Geometry: final body of the model. Coordinates: model frame, mm. A direction names the side the tool comes from. Round coordinates to 2 decimals unless told otherwise and drop trailing zeros. Loops run counter-clockwise (first coordinate to the right, second up) from the corner with the lowest first, then second, coordinate; pieces in that order, holes last. Notation, with made-up numbers: (-31, 37.5) -> (21, 37.5) arc R15 ccw to (21, 61.5) -> close; hole circle Ø3 at (29.5, -12). An arc over 180 degrees is marked (long way). Answer in a Markdown table with one row per item.
```python
from build123d import *

# Parameters (mm, degrees)
F0_R     = 35
F0_R_2   = 32.5
F1_DEPTH = 40
F2_START = 20
F0_R_3   = 12.5
F2_DEPTH = 20
F3_START = 39
F3_DEPTH = 61
F4_SIZE  = 20
F5_SIZE  = 18.99999
F6_START = 3
F0_R_4   = 40
F6_DEPTH = 12
F7_SIZE  = 4.99999
F8_DEPTH = 1.5


# Not quite as in the source:
# - a fillet or chamfer is up to 0.001 mm smaller than in the source, because OpenCascade refuses the exact size


with BuildPart() as f1:
    # F0 (on Top) → F1 (new body)
    with BuildSketch(Plane.XY):
        Circle(F0_R)
        Circle(F0_R_2, mode=Mode.SUBTRACT)
    extrude(amount=F1_DEPTH)

    # F0 (on Top) → F2 (join)
    with BuildSketch(Plane.XY.offset(F2_START)):
        Circle(F0_R_2)
        Circle(F0_R_3, mode=Mode.SUBTRACT)
    extrude(amount=F2_DEPTH)

    # F0 (on Top) → F3 (join)
    with BuildSketch(Plane.XY.offset(F3_START)):
        Circle(F0_R_3)
    extrude(amount=F3_DEPTH)

    # F4
    f4_edges = [f1.edges().sort_by_distance(p)[0] for p in [
        (-35, 0, 40),
    ]]
    chamfer(f4_edges, length=F4_SIZE)

    # F5 (size 19 in the source; OpenCascade refuses exactly that, so slightly less here)
    f5_edges = [f1.edges().sort_by_distance(p)[0] for p in [
        (-12.5, 0, 20),
    ]]
    chamfer(f5_edges, length=F5_SIZE)

    # F0 (on Top) → F6 (join)
    with BuildSketch(Plane.XY.offset(F6_START)):
        Circle(F0_R_4)
        Circle(F0_R, mode=Mode.SUBTRACT)
    extrude(amount=F6_DEPTH)

    # F7 (size 5 in the source; OpenCascade refuses exactly that, so slightly less here)
    f7_edges = [f1.edges().sort_by_distance(p)[0] for p in [
        (-40, 0, 3),
        (-40, 0, 15),
    ]]
    chamfer(f7_edges, length=F7_SIZE)

    # F8 (cut): a face of the model
    f8_faces = [f1.faces().sort_by_distance(p)[0] for p in [
        (-34.0100505063, 0, 0),
    ]]
    extrude(f8_faces, amount=-F8_DEPTH, mode=Mode.SUBTRACT)


solid = f1.part
```
Item 1: Set-up query: faces 1 (the cylindrical face through (31, 9.76, 10.62)), 2 (the flat face through (0, 0, 100)), 3 (the flat face through (-3.4, 12.3, 40)). Return all of +Z, -Z, +X, -X, +Y, -Y with unobstructed straight access to the full face (end or side cutting, diameter ignored); none if empty.
Ans:
| item | result |
|---|---|
| face 1 | -Z |
| face 2 | +Z, +X, -X, +Y, -Y |
| face 3 | +Z |
Item 2: Mould query, pull axis Y, two halves, no side actions, for faces 4 (the flat face through (23.2, -23.2, 1.5)), 5 (the flat face through (-17, 27, 20)), 6 (the conical face through (33.615, 10.586, 14.757)). Classes: released by +Y, released by -Y, zero draft, split by the parting line, or undercut.
Ans:
| item | result |
|---|---|
| face 4 | zero draft |
| face 5 | undercut |
| face 6 | split by the parting line |
Item 3: Section query C-C, the plane z = 59.5. Output: boundary loops of the cut face in (x, y), and give its area (3 significant figures).
Ans:
| item | result |
|---|---|
| outline | circle Ø25 at (0, 0) |
| area | 491 mm2 |
Item 4: Ray query, L1, parallel to Y at x = 0, z = 15; L2, parallel to Y at x = -3.5, z = 23; L3, parallel to Z at x = 6, y = -5. Return the intervals inside material, ascending.
Ans:
| item | result |
|---|---|
| L1 | -35 to -32.5, 32.5 to 35 |
| L2 | -31.81 to -28.28, 28.28 to 31.81 |
| L3 | 39 to 100 |
Item 5: First-contact query: P1, Ø19.5, axis at x = 2, y = -3.5, coming from the -Z side; P2, Ø6, axis at y = 19.5, z = 14, coming from the -X side; P3, Ø7.5, axis at x = -3, y = 0.5, coming from the -Z side. Flat tips, straight axial feed; report the tip coordinate or a pass-through.
Ans:
| item | result |
|---|---|
| P1 | z = 37.72 |
| P2 | x = -34.16 |
| P3 | z = 39 |
